```python
from build123d import *

# Parameters (mm, degrees)
SKETCH1_R           = 200
BOSS_EXTRUDE1_DEPTH = 100
CUT_EXTRUDE2_DEPTH  = 100
BOSS_EXTRUDE2_DEPTH = 75.993421
BOSS_EXTRUDE3_DEPTH = 75.993421
SKETCH9_R           = 159.375
BOSS_EXTRUDE4_DEPTH = 151.986842
CUT_EXTRUDE3_START  = -60
SKETCH11_R          = 159.375
CUT_EXTRUDE3_DEPTH  = 60
CUT_EXTRUDE4_DEPTH  = 5
CUT_EXTRUDE5_DEPTH  = 5
SKETCH15_R          = 132.8125
BOSS_EXTRUDE5_DEPTH = 10
SKETCH16_R          = 132.8125
BOSS_EXTRUDE6_DEPTH = 10


with BuildPart() as part:
    # Sketch1 → Boss-Extrude1 (new body)
    with BuildSketch(Plane(origin=(0, 0, 0), x_dir=(1, 0, 0), z_dir=(0, 1, 0))):
        with Locations(Location((0, 0, 0), (0, 0, 270))):
            Circle(SKETCH1_R)
    extrude(amount=BOSS_EXTRUDE1_DEPTH)

    # Sketch2 → Cut-Extrude2 (cut)
    with BuildSketch(Plane(origin=(0, 100, 0), x_dir=(1, 0, 0), z_dir=(0, 1, 0))):
        Polygon((185, 0), (185, 120.642549135), (200, 120.642549135), (200, 0), (200, -137.849885779), (185, -137.849885779), align=None)
    extrude(amount=-CUT_EXTRUDE2_DEPTH, mode=Mode.SUBTRACT)

    # Sketch4 → Boss-Extrude2 (add)
    with BuildSketch(Plane.XY):
        Polygon((185, 50), (185, 0), (0, 0), (251.924557131, -112.966443103), (387.075695624, -112.966443103), align=None)
    extrude(amount=-BOSS_EXTRUDE2_DEPTH)

    # Sketch7 → Boss-Extrude3 (add)
    with BuildSketch(Plane.XY):
        Polygon((0, 0), (185, 0), (185, 50), (387.075695624, -112.966443103), (251.924557131, -112.966443103), align=None)
    extrude(amount=BOSS_EXTRUDE3_DEPTH)

    # Sketch9 → Boss-Extrude4 (add)
    with BuildSketch(Plane.XY.offset(75.993420768)):
        with Locations((387.075695624, -112.966443103)):
            Circle(SKETCH9_R)
    extrude(amount=-BOSS_EXTRUDE4_DEPTH)

    # Sketch11 → Cut-Extrude3 (cut)
    with BuildSketch(Plane(origin=(0, 0, -75.993420768), x_dir=(-1, 0, 0), z_dir=(0, 0, -1)).offset(CUT_EXTRUDE3_START)):
        with Locations((-387.075695624, -112.966443103)):
            Circle(SKETCH11_R)
    extrude(amount=CUT_EXTRUDE3_DEPTH, mode=Mode.SUBTRACT)


with BuildPart() as cut_extrude3_kept_piece:
    # of the separate pieces the step leaves, the one the design keeps (cut_extrude3_pieces_kept)
    add(part.part.solids().sort_by_distance((185, 0, -75.993420884))[0])

    # Sketch12 → Cut-Extrude4 (cut)
    with BuildSketch(Plane.XY.offset(75.993420768)):
        with BuildLine():
            Line((185, 0), (0, 0))
            Line((0, 0), (228.060355378, -102.265406172))
            ThreePointArc((228.060355378, -102.265406172), (238.589276077, -54.846272892), (262.770904395, -12.719307371))
            Line((262.770904395, -12.719307371), (185, 50))
            Line((185, 50), (185, 0))
        make_face()
    extrude(amount=-CUT_EXTRUDE4_DEPTH, mode=Mode.SUBTRACT)

    # Sketch14 → Cut-Extrude5 (cut)
    with BuildSketch(Plane(origin=(0, 0, -75.993420768), x_dir=(-1, 0, 0), z_dir=(0, 0, -1))):
        with BuildLine():
            Line((-228.060355378, -102.265406172), (0, 0))
            Line((0, 0), (-185, 0))
            Line((-185, 0), (-185, 50))
            Line((-185, 50), (-263.016769179, -12.917588066))
            ThreePointArc((-263.016769179, -12.917588066), (-238.655621962, -54.898617596), (-228.060355378, -102.265406172))
        make_face()
    extrude(amount=-CUT_EXTRUDE5_DEPTH, mode=Mode.SUBTRACT)

    # Sketch15 → Boss-Extrude5 (add)
    with BuildSketch(Plane(origin=(0, 0, -15.993420768), x_dir=(-1, 0, 0), z_dir=(0, 0, -1))):
        with Locations((-387.075695624, -112.966443103)):
            Circle(SKETCH15_R)
    extrude(amount=BOSS_EXTRUDE5_DEPTH)

    # Sketch16 → Boss-Extrude6 (add)
    with BuildSketch(Plane(origin=(0, 100, 0), x_dir=(1, 0, 0), z_dir=(0, 1, 0))):
        with Locations(Location((0, 0, 0), (0, 0, 270))):
            Circle(SKETCH16_R)
    extrude(amount=BOSS_EXTRUDE6_DEPTH)


solid = cut_extrude3_kept_piece.part
```
Input: part model. Units: mm. Frame: model coordinates. A direction names the side the tool comes from. Give positions to 0.01 mm unless a question says otherwise; leave off trailing zeros. Write each loop counter-clockwise with the first axis right and the second up, starting at its lowest first coordinate (ties: lowest second). Pieces come first, ordered by that corner, then holes. Notation, with made-up numbers: (10, -36.5) - (31, -36.5) arc R6 cw to (31, -26.5) - close; hole circle Ø10 at (12.25, -7). An arc over 180 degrees is marked (long way). Write item = value, one per line. Start each with the question number.
1) Cut plane C-C (y = -198). Return loops of the section in (x, z).
2) Cut plane D-D (z = -109). Return loops of the section in (x, y), and give its area (3 significant figures).
3) Draft query along X for faces 4 (the face through (238.344, -55.483, 73.528)), 5 (the face through (-133, 100, -3)), 6 (the face through (260.396, -73.073, -20.923)), 7 (the face through (223.462, 18.982, 1.471)). Return one class per face: pulls with the +X half, pulls with the -X half, needs draft (parallel to the pull), parting line crosses it, or undercut.
4) Pin query (flat end, axial travel): pin 1 (2 mm diameter, centred on x = 351, y = 1, fed in from +Z); pin 2 (12 mm diameter, centred on y = 12, z = -38, fed in from -X); pin 3 (1.5 mm diameter, centred on x = -26, z = 134, fed in from +Y). Return the tip coordinate at first contact, or that it passes through.
5) Cut plane B-B (x = 71.5). Return loops of the section in (y, z).
6) Reachability of faces 1 (the face through (447, 6, -15.993)), 2 (the face through (39.89, 104.93, 126.68)), 3 (the face through (-48, 0, -3)) from +Z, -Z, +X, -X, +Y, -Y: full face, straight path, thin tool, end or side. Return the list, or none.
7) Material intervals for L1, parallel to Y at x = -37, z = 69.5; L2, parallel to X at y = 69.5, z = 2.5; L3, parallel to Y at x = -122, z = 134.5, sorted ascending. Write a range as [from, to].
Answers follow:
q1.outline = (252.28, -15.99) - (285.05, -15.99) - (285.05, -25.99) - (489.1, -25.99) - (489.1, -15.99) - (521.87, -15.99) - (521.87, 75.99) - (252.28, 75.99) - close
q2.outline = (-167.69, 0) - (167.69, 0) - (167.69, 100) - (75.88, 100) - (75.88, 110) - (-75.88, 110) - (-75.88, 100) - (-167.69, 100) - close
q2.area = 35,100 mm^2
q3.face_4 = pulls with the -X half
q3.face_5 = needs draft
q3.face_6 = undercut
q3.face_7 = undercut
q4.pin_1 = 75.99
q4.pin_2 = -197.42
q4.pin_3 = 100
q5.outline = (-32.06, -70.99) - (0, -70.99) - (0, -186.78) - (100, -186.78) - (100, -111.92) - (110, -111.92) - (110, 111.92) - (100, 111.92) - (100, 186.78) - (0, 186.78) - (0, 70.99) - (-32.06, 70.99) - close
q6.face_1 = -Z
q6.face_2 = +Y
q6.face_3 = -X, -Y
q7.L1 = [0, 110]
q7.L2 = [-199.98, 185]
q7.L3 = [0, 100]
